The drawing under review shows one solid part. Ordinate dimensions are in mm from its lowest x, y, z. Give positions to 0.01 mm unless a question says otherwise; leave off trailing zeros. Loops run counter-clockwise (first coordinate to the right, second up) from the corner with the lowest first, then second, coordinate; pieces in that order, holes last. Notation, with made-up numbers: M 79,83 L 89,83 A23 ccw 89,106 Z; hole C 6,32 d7. An arc over 180 degrees is marked long. One line per item, written item: value. Start each with the question number.
Q1. Mouldability with a two-part tool opening along Z and no side actions: class the marked faces 1, 2, 3 and 4 as released by +Z, released by -Z, zero draft, split by the parting line, or undercut.
Q2. To check wall thickness, follow line 1 along Z through (x, y) = (2.5, 1.65); line 2 along X through (y, z) = (0.7, 2.5); line 3 along Z through (x, y) = (3.5, 2.5). State the ranges of each line that lie inside material, in increasing order. Write a range as from..to.
Q3. We need section A-A on y = 2.6. Write out the cut boundary in (x, z).
Q4. We need section B-B on z = 3.5. Write out the cut boundary in (x, y), plus the area to 3 significant figures.
Q5. We need section C-C on x = 24.13. Write out the cut boundary in (y, z).
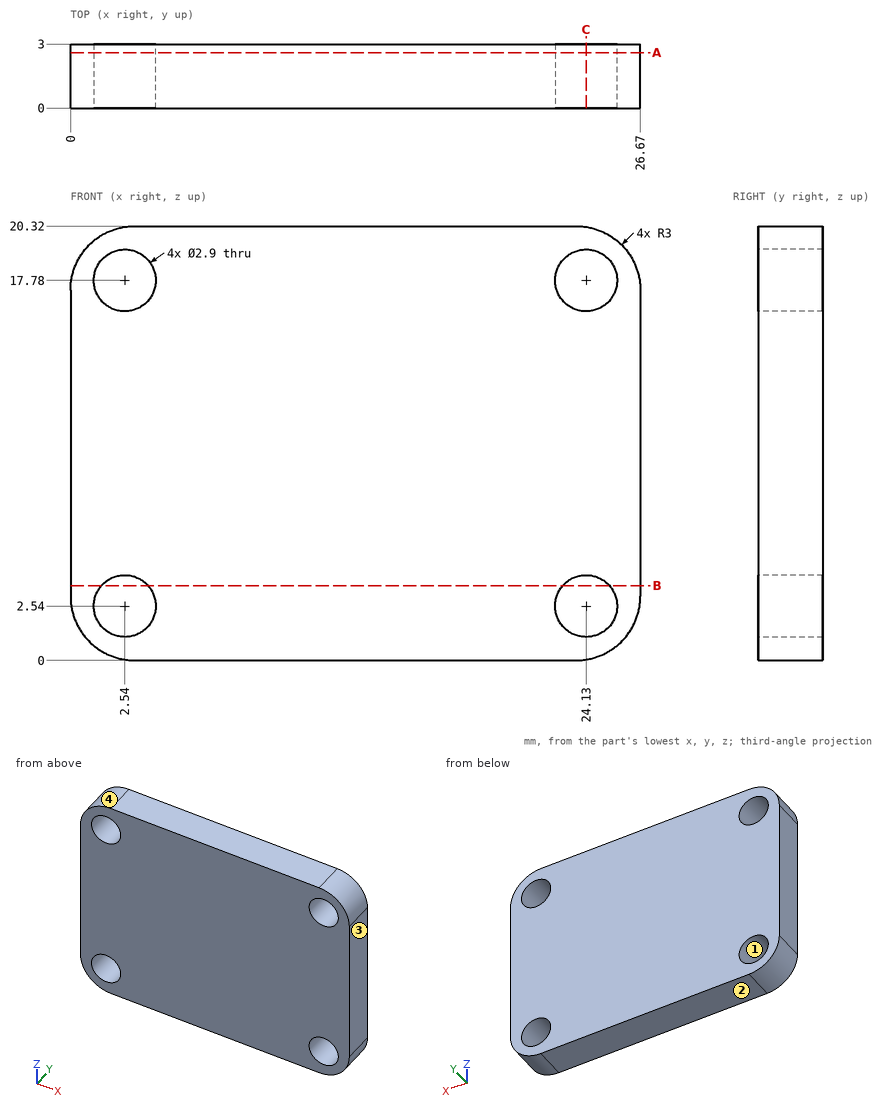
Solved:
1. face 1: undercut
1. face 2: released by -Z
1. face 3: zero draft
1. face 4: released by +Z
2. line 1: 0.04..1.09, 3.99..16.33, 19.23..20.28
2. line 2: 0.04..1.09, 3.99..22.68, 25.58..26.63
2. line 3: 0..1.45, 3.63..16.69, 18.87..20.32
3. outline: M 0,3 A3 ccw 3,0 L 23.67,0 A3 ccw 26.67,3 L 26.67,17.32 A3 ccw 23.67,20.32 L 3,20.32 A3 ccw 0,17.32 Z; hole C 2.54,2.54 d2.9; hole C 2.54,17.78 d2.9; hole C 24.13,2.54 d2.9; hole C 24.13,17.78 d2.9
4. outline: M 0,0 L 1.45,0 L 1.45,3 L 0,3 Z; M 3.63,0 L 23.04,0 L 23.04,3 L 3.63,3 Z; M 25.22,0 L 26.67,0 L 26.67,3 L 25.22,3 Z
4. area: 67.0 mm2
5. outline: M 0,0.04 L 3,0.04 L 3,1.09 L 0,1.09 Z; M 0,3.99 L 3,3.99 L 3,16.33 L 0,16.33 Z; M 0,19.23 L 3,19.23 L 3,20.28 L 0,20.28 Z
